Input: part model. Units: mm. Frame: model coordinates. A direction names the side the tool comes from. Give positions to 0.01 mm unless a question says otherwise; leave off trailing zeros. Loops run counter-clockwise (first coordinate to the right, second up) from the corner with the lowest first, then second, coordinate; pieces in that order, holes last. Notation, with made-up numbers: (43, 66.25) - (68, 66.25) arc R30 cw to (68, 92.25) - close; hole circle Ø9 at (19.25, -6.5). An arc over 180 degrees is marked (long way). Answer as a JSON object with one key per item and string values.
from build123d import *

# Parameters (mm, degrees)
F1_DEPTH = 200


# Not quite as in the source:
# - ends of sketch curves that miss each other by under 0.0002 mm in the source are joined


with BuildPart() as f1:
    # F0 (on Front) → F1 (new body)
    with BuildSketch(Plane.XZ):
        with BuildLine():
            Line((26.171612, -51.228388), (28, -52.5))
            Line((28, -52.5), (30, -52.5))
            Line((30, -52.5), (30, 16.5))
            ThreePointArc((30, 16.5), (29.4142135624, 17.9142135624), (28, 18.5))
            Line((28, 18.5), (22, 18.5))
            Line((22, 18.5), (22, 17.5))
            Line((22, 17.5), (20, 17.5))
            Line((20, 17.5), (20, 14.5))
            Line((20, 14.5), (22, 14.5))
            Line((22, 14.5), (22, 11.643728))
            ThreePointArc((22, 11.643728), (22.746864, 10.896864), (23.493728, 11.643728))
            ThreePointArc((23.493728, 11.643728), (26.310454189, 12.810454189), (25.143728, 9.993728))
            ThreePointArc((25.143728, 9.993728), (24.396864, 9.246864), (25.143728, 8.5))
            Line((25.143728, 8.5), (26.5, 8.5))
            Line((26.5, 8.5), (26.5, 4.5))
            Line((26.5, 4.5), (23.5, 4.5))
            Line((23.5, 4.5), (23.5, 2.5))
            Line((23.5, 2.5), (25.5, 2.5))
            Line((25.5, 2.5), (25.5, 0))
            Line((25.5, 0), (18.5, 0))
            Line((18.5, 0), (18.5, 2.5))
            Line((18.5, 2.5), (20.5, 2.5))
            Line((20.5, 2.5), (20.5, 4.5))
            Line((20.5, 4.5), (12.5, 4.5))
            Line((12.5, 4.5), (12.5, 2.5))
            Line((12.5, 2.5), (14.5, 2.5))
            Line((14.5, 2.5), (14.5, 0))
            Line((14.5, 0), (7.5, 0))
            Line((7.5, 0), (7.5, 2.5))
            Line((7.5, 2.5), (9.5, 2.5))
            Line((9.5, 2.5), (9.5, 4.5))
            Line((9.5, 4.5), (1.5, 4.5))
            Line((1.5, 4.5), (1.5, 2.5))
            Line((1.5, 2.5), (3.5, 2.5))
            Line((3.5, 2.5), (3.5, 0))
            Line((3.5, 0), (-3.5, 0))
            Line((-3.5, 0), (-3.5, 2.5))
            Line((-3.5, 2.5), (-1.5, 2.5))
            Line((-1.5, 2.5), (-1.5, 4.5))
            Line((-1.5, 4.5), (-9.5, 4.5))
            Line((-9.5, 4.5), (-9.5, 2.5))
            Line((-9.5, 2.5), (-7.5, 2.5))
            Line((-7.5, 2.5), (-7.5, 0))
            Line((-7.5, 0), (-14.5, 0))
            Line((-14.5, 0), (-14.5, 2.5))
            Line((-14.5, 2.5), (-12.5, 2.5))
            Line((-12.5, 2.5), (-12.5, 4.5))
            Line((-12.5, 4.5), (-20.5, 4.5))
            Line((-20.5, 4.5), (-20.5, 2.5))
            Line((-20.5, 2.5), (-18.5, 2.5))
            Line((-18.5, 2.5), (-18.5, 0))
            Line((-18.5, 0), (-25.5, 0))
            Line((-25.5, 0), (-25.5, 2.5))
            Line((-25.5, 2.5), (-23.5, 2.5))
            Line((-23.5, 2.5), (-23.5, 4.5))
            Line((-23.5, 4.5), (-26.5, 4.5))
            Line((-26.5, 4.5), (-26.5, 8.5))
            Line((-26.5, 8.5), (-25.143728, 8.5))
            ThreePointArc((-25.143728, 8.5), (-24.396864, 9.246864), (-25.143728, 9.993728))
            ThreePointArc((-25.143728, 9.993728), (-26.310454189, 12.810454189), (-23.493728, 11.643728))
            ThreePointArc((-23.493728, 11.643728), (-22.746864, 10.896864), (-22, 11.643728))
            Line((-22, 11.643728), (-22, 14.5))
            Line((-22, 14.5), (-20, 14.5))
            Line((-20, 14.5), (-20, 17.5))
            Line((-20, 17.5), (-22, 17.5))
            Line((-22, 17.5), (-22, 18.5))
            Line((-22, 18.5), (-28, 18.5))
            ThreePointArc((-28, 18.5), (-29.4142135624, 17.9142135624), (-30, 16.5))
            Line((-30, 16.5), (-30, -52.5))
            Line((-30, -52.5), (-28, -52.5))
            Line((-28, -52.5), (-26.171612, -51.228388))
            ThreePointArc((-26.171612, -51.228388), (-26.0454895845, -51.0852629626), (-26, -50.9))
            ThreePointArc((-26, -50.9), (-26.1171572875, -50.6171572875), (-26.4, -50.5))
            Line((-26.4, -50.5), (-28, -50.5))
            Line((-28, -50.5), (-28, -48.5))
            Line((-28, -48.5), (28, -48.5))
            Line((28, -48.5), (28, -50.5))
            Line((28, -50.5), (26.4, -50.5))
            ThreePointArc((26.4, -50.5), (26.1171572875, -50.6171572875), (26, -50.9))
            ThreePointArc((26, -50.9), (26.0454895845, -51.0852629626), (26.171612, -51.228388))
        make_face()
        with BuildLine():
            Line((-22, -46.5), (-22, -41.643728))
            ThreePointArc((-22, -41.643728), (-22.746864, -40.896864), (-23.493728, -41.643728))
            ThreePointArc((-23.493728, -41.643728), (-26.310454189, -42.810454189), (-25.143728, -39.993728))
            ThreePointArc((-25.143728, -39.993728), (-24.396864, -39.246864), (-25.143728, -38.5))
            Line((-25.143728, -38.5), (-28, -38.5))
            Line((-28, -38.5), (-28, -36.5))
            Line((-28, -36.5), (-25, -36.5))
            Line((-25, -36.5), (-25, -34.5))
            Line((-25, -34.5), (-28.5, -34.5))
            Line((-28.5, -34.5), (-28.5, -1.5))
            Line((-28.5, -1.5), (28.5, -1.5))
            Line((28.5, -1.5), (28.5, -34.5))
            Line((28.5, -34.5), (25, -34.5))
            Line((25, -34.5), (25, -36.5))
            Line((25, -36.5), (28, -36.5))
            Line((28, -36.5), (28, -38.5))
            Line((28, -38.5), (25.143728, -38.5))
            ThreePointArc((25.143728, -38.5), (24.396864, -39.246864), (25.143728, -39.993728))
            ThreePointArc((25.143728, -39.993728), (26.310454189, -42.810454189), (23.493728, -41.643728))
            ThreePointArc((23.493728, -41.643728), (22.746864, -40.896864), (22, -41.643728))
            Line((22, -41.643728), (22, -46.5))
            Line((22, -46.5), (-22, -46.5))
        make_face(mode=Mode.SUBTRACT)
    extrude(amount=F1_DEPTH)


solid = f1.part
Item 1: Access query for faces 1 (the face through (11, -99, 0)), 2 (the face through (6, -99, 4.5)), 3 (the face through (0, -200, -1)). Directions: +Z, -Z, +X, -X, +Y, -Y. A direction counts if a zero-diameter tool reaches every point of the face in a straight line with its end or side. Return the directions, or none.
Geometry check:
{"face 1": "+Y, -Y", "face 2": "+Z, +Y, -Y", "face 3": "+Z, -Z, +X, -X, -Y"}
Item 2: Mould query, pull axis X, two halves, no side actions, for faces 4 (the face through (0, 0, -1)), 5 (the face through (30, -99, -18)), 6 (the face through (-11, -99, 0)). Classes: released by +X, released by -X, zero draft, split by the parting line, or undercut.
Geometry check:
{"face 4": "zero draft", "face 5": "released by +X", "face 6": "undercut"}
Item 3: Cut plane A-A (z = -5.5). Return loops of the section in (x, y), then the cut area to 3 significant figures.
Geometry check:
{"outline": "(-30, -200) - (-28.5, -200) - (-28.5, 0) - (-30, 0) - close; (28.5, -200) - (30, -200) - (30, 0) - (28.5, 0) - close", "area": "600 mm2"}
Item 4: Contact query for flat-ended pins moving along their axis: P1, Ø1.1, axis at x = 26, y = -80.5, coming from the -Z side; P2, Ø6, axis at x = -2, y = -131.5, coming from the -Z side; P3, Ø6, axis at x = -9.5, y = -98, coming from the +Z side; P4, Ø3, axis at x = 25.14, z = 11.64, coming from the -Y side. Output: stop coordinate, or through.
Geometry check:
{"P1": "stops at z = -51.49", "P2": "stops at z = -48.5", "P3": "stops at z = 4.5", "P4": "passes through"}
Item 5: Material intervals for line 1 (Z direction, x = 2.5, y = -118); line 2 (Z direction, x = 23, y = -130.5); line 3 (X direction, y = -49.5, z = -11), sorted ascending. Write a range as [from, to].
Geometry check:
{"line 1": "z = [-48.5, -46.5], [-1.5, 0], [2.5, 4.5]", "line 2": "z = [-48.5, -40.94], [-1.5, 0], [10.94, 18.5]", "line 3": "x = [-30, -28.5], [28.5, 30]"}
